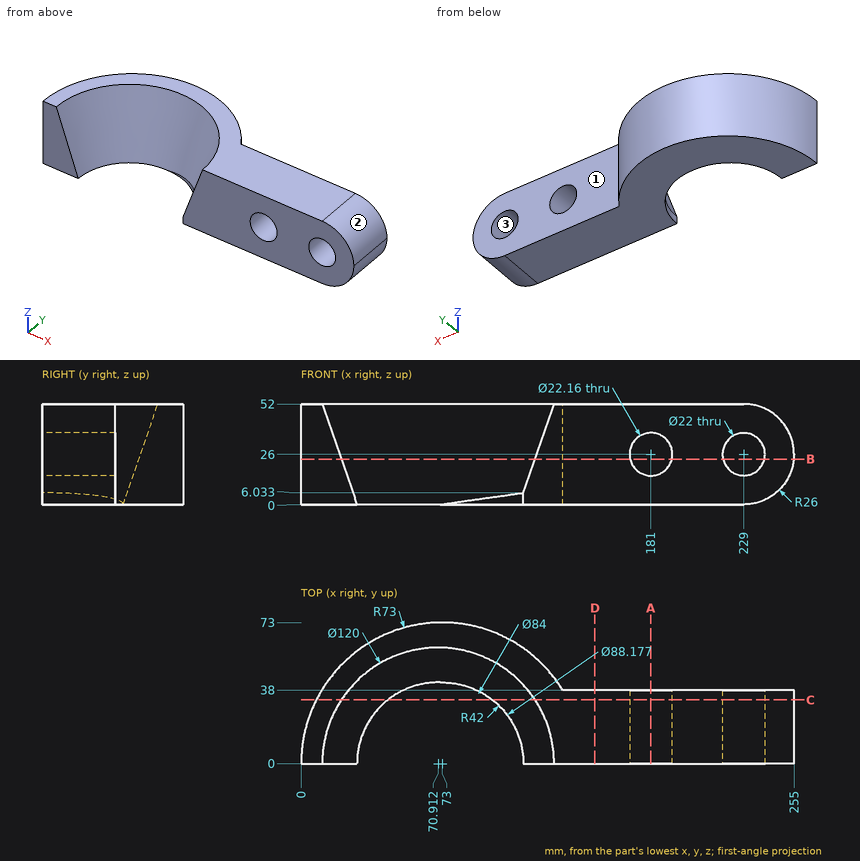
Could you check a few things on this drawing? It's one solid part, dimensions in mm from its lowest x, y, z. Coordinates: 2 decimals unless noted, no trailing zeros. Order: outer loops, then holes, each group sorted by start corner. A loop starts at its lowest first (then second) coordinate and runs counter-clockwise, first axis right, second up. Notation, with made-up numbers: (-34.75, 16) -> (-8.75, 16) arc R36 ccw to (-8.75, 53) -> close; hole circle Ø9 at (-3, 18.5). An arc over 180 degrees is marked (long way). Answer in a Markdown table with one row per item.
(1) Please list where these lines run through material, in increasing order: probe 1 along Z at (x, y) = (181, 20); probe 2 along X at (y, z) = (14, 29.5) (1 decimal); probe 3 along Y at (x, z) = (220.5, 10.5).
Answer key:
| item | result |
|---|---|
| probe 1 | 0 to 14.92, 37.08 to 52 |
| probe 2 | 1.4 to 20.6, 121.2 to 170.5, 191.5 to 218.6, 239.4 to 254.8 |
| probe 3 | 0 to 38 |
(2) Thinking about a two-plate mould opening in Z: for the marked faces 1, 2 and 3, which applies, +Z half, -Z half, draft (parallel to the pull), parting line (faces both ways), or undercut?
Answer key:
| item | result |
|---|---|
| face 1 | draft |
| face 2 | +Z half |
| face 3 | undercut |
(3) I want a section at C-C on y = 33. Count the separate pieces of the cut face and the enclosed holes in it, then the cut area to 3 significant figures.
Answer key:
| item | result |
|---|---|
| separate pieces | 2 |
| enclosed holes | 2 |
| area | 7,770 mm^2 |
(4) I want a section at D-D on x = 152. List the corners of the cut face in (y, z) for me, then the cut area to 3 significant figures.
Answer key:
| item | result |
|---|---|
| outline | (0, 0) -> (38, 0) -> (38, 52) -> (0, 52) -> close |
| area | 1,980 mm^2 |
(5) I want a section at B-B on z = 23.5. List the corners of the cut face in (x, y) for me (1 decimal), then the cut area to 3 significant figures.
Answer key:
| item | result |
|---|---|
| outline | (0, 0) -> (20.8, 0) arc R50.1 cw to (121, 0) -> (170.2, 0) -> (170.2, 38) -> (135.3, 38) arc R73 ccw to start; (191.8, 0) -> (218.3, 0) -> (218.3, 38) -> (191.8, 38) -> close; (239.7, 0) -> (254.9, 0) -> (254.9, 38) -> (239.7, 38) -> close |
| area | 7,060 mm^2 |
(6) Will these pins go through, and if not, where does the flat tip stop? pin 1 Ø1 at (x, z) = (48.5, 29) entering from -Y; pin 2 Ø13 at (x, z) = (229, 26) entering from +Y; pin 3 Ø15.5 at (x, z) = (207.5, 29.5) entering from +Y; pin 4 Ø1 at (y, z) = (43, 7.5) entering from -X.
Answer key:
| item | result |
|---|---|
| pin 1 | y = 46.66 |
| pin 2 | through |
| pin 3 | y = 38 |
| pin 4 | x = 13.65 |
(7) I want a section at A-A on x = 181. List the corners of the cut face in (y, z) for me.
Answer key:
| item | result |
|---|---|
| outline | (0, 0) -> (38, 0) -> (38, 14.92) -> (0, 14.92) -> close; (0, 37.08) -> (38, 37.08) -> (38, 52) -> (0, 52) -> close |
